```python
from build123d import *

# Parameters (mm, degrees)
F1_DEPTH  = 78.74
F4_W      = 50.8
F4_H      = 25.4
F6_DEPTH  = 11.43
F7_W      = 48.6228571429
F7_H      = 23.7671428571
F10_DEPTH = 3.81
F12_DEPTH = 53.34
F14_DEPTH = 38.1
F16_D     = 6.7564
F16_DEPTH = 7.62
F16_TIP   = 2.0298273432


with BuildPart() as f1:
    # F0 (on Front) → F1 (new body)
    with BuildSketch(Plane.XZ):
        with BuildLine():
            Line((-21.59, 12.7), (-21.59, -12.7))
            ThreePointArc((-21.59, -12.7), (0, -34.29), (21.59, -12.7))
            Line((21.59, -12.7), (21.59, 0))
            Line((21.59, 0), (21.59, 12.7))
            ThreePointArc((21.59, 12.7), (0, 34.29), (-21.59, 12.7))
        make_face()
    extrude(amount=F1_DEPTH)

    # F4 (on Front) → F5 section 0
    with BuildSketch(Plane.XZ):
        with BuildLine():
            Line((-25.4, 12.7), (25.4, 12.7))
            ThreePointArc((25.4, 12.7), (0, 38.1), (-25.4, 12.7))
        make_face()
    # F3 (on offset) → F5 section 1
    with BuildSketch(Plane.XZ.offset(-26.67)):
        with BuildLine():
            Line((-22.86, 8.89), (22.86, 8.89))
            ThreePointArc((22.86, 8.89), (0, 31.75), (-22.86, 8.89))
        make_face()
    loft()

    # F4 (on Front) → F6 (join)
    with BuildSketch(Plane.XZ):
        with BuildLine():
            Line((-25.4, 12.7), (25.4, 12.7))
            ThreePointArc((25.4, 12.7), (0, 38.1), (-25.4, 12.7))
        make_face()
        Rectangle(F4_W, F4_H)
        with BuildLine():
            ThreePointArc((-25.4, -12.7), (0, -38.1), (25.4, -12.7))
            Line((25.4, -12.7), (-25.4, -12.7))
        make_face()
    extrude(amount=-F6_DEPTH)

    # F7 (on face) → F8 section 0
    with BuildSketch(Plane(origin=(0, 11.43, 0), x_dir=(-1, 0, 0), z_dir=(0, 1, 0))):
        with Locations((0, -0.8164285714)):
            Rectangle(F7_W, F7_H)
    # F3 (on offset) → F8 section 1
    with BuildSketch(Plane.XZ.offset(-26.67)):
        with BuildLine():
            ThreePointArc((22.7188888889, 6.3539227823), (22.8246949596, 7.62), (22.86, 8.89))
            Line((22.86, 8.89), (-22.86, 8.89))
            ThreePointArc((-22.86, 8.89), (-22.8245852305, 7.61802946), (-22.7184506514, 6.35))
            Line((-22.7184506514, 6.35), (22.7188888889, 6.3539227823))
        make_face()
    loft()

    # F3 (on offset) → F9 section 0
    with BuildSketch(Plane.XZ.offset(-26.67)):
        with BuildLine():
            ThreePointArc((-22.7184506514, 6.35), (0.0019735927, -13.9699999148), (22.7188888889, 6.3539227823))
            Line((22.7188888889, 6.3539227823), (-22.7184506514, 6.35))
        make_face()
    # F7 (on face) → F9 section 1
    with BuildSketch(Plane(origin=(0, 11.43, 0), x_dir=(-1, 0, 0), z_dir=(0, 1, 0))):
        with BuildLine():
            Line((24.3114285714, -12.7), (-24.3114285714, -12.7))
            ThreePointArc((-24.3114285714, -12.7), (0, -37.0114285714), (24.3114285714, -12.7))
        make_face()
    loft()

    # F3 (on offset) → F10 (join)
    with BuildSketch(Plane.XZ.offset(-26.67)):
        with BuildLine():
            Line((-22.86, 8.89), (22.86, 8.89))
            ThreePointArc((22.86, 8.89), (0, 31.75), (-22.86, 8.89))
        make_face()
        with BuildLine():
            ThreePointArc((22.7188888889, 6.3539227823), (22.8246949596, 7.62), (22.86, 8.89))
            Line((22.86, 8.89), (-22.86, 8.89))
            ThreePointArc((-22.86, 8.89), (-22.8245852305, 7.61802946), (-22.7184506514, 6.35))
            Line((-22.7184506514, 6.35), (22.7188888889, 6.3539227823))
        make_face()
        with BuildLine():
            ThreePointArc((-22.7184506514, 6.35), (0.0019735927, -13.9699999148), (22.7188888889, 6.3539227823))
            Line((22.7188888889, 6.3539227823), (-22.7184506514, 6.35))
        make_face()
    extrude(amount=-F10_DEPTH)

    # F11 (on Front) → F12 (join)
    with BuildSketch(Plane.XZ):
        with BuildLine():
            Line((12.7, 12.7), (12.7, 34.6970452561))
            ThreePointArc((12.7, 34.6970452561), (0, 38.1), (-12.7, 34.6970452561))
            Line((-12.7, 34.6970452561), (-12.7, 12.7))
            Line((-12.7, 12.7), (12.7, 12.7))
        make_face()
    extrude(amount=F12_DEPTH)

    # F13 (on Top) → F14 (join)
    with BuildSketch(Plane.XY):
        Polygon((21.59, -35.56), (21.59, 15.24), (-21.59, 15.24), (-21.59, -35.56), (-8.89, -35.56), (-8.89, -78.74), (8.89, -78.74), (8.89, -35.56), align=None)
    extrude(amount=-F14_DEPTH)

    # F16
    with Locations(Plane(origin=(0, 0, -38.1), x_dir=(1, 0, 0), z_dir=(0, 0, -1))):
        with Locations((0, 55.88)):
            Hole(F16_D / 2, depth=F16_DEPTH)
            with Locations((0, 0, -(F16_DEPTH + F16_TIP / 2))):  # 118° drill point
                Cone(0, F16_D / 2, F16_TIP, mode=Mode.SUBTRACT)


solid = f1.part
```
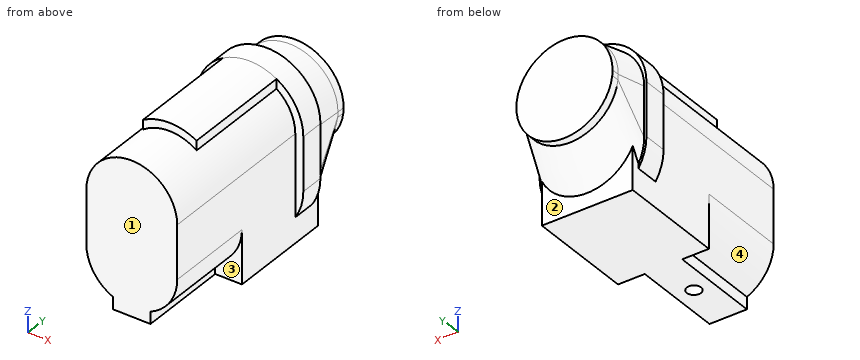
Check sheet for the modelled part. Datum: model origin and axes. Units: mm. Face numbers are marked on the shaded views. A direction names the side the tool comes from. Coordinates: 2 decimals unless noted, no trailing zeros. Write each loop counter-clockwise with the first axis right and the second up, starting at its lowest first coordinate (ties: lowest second). Pieces come first, ordered by that corner, then holes. Notation, with made-up numbers: (42, 1.5) - (59, 1.5) arc R22 ccw to (59, 7.5) - close; hole circle Ø9 at (62.5, 24.5). An arc over 180 degrees is marked (long way). One line per question, with ' | ' between items.
Item 1: Access from +Z, -Z, +X, -X, +Y, -Y to the whole of each face (thin tool, end or side, straight path). Record for the marked faces 1, 2, 3 and 4.
Determined:
face 1: +Z, -Z, +X, -X, -Y | face 2: -Z, +Y | face 3: -Z, +X, -Y | face 4: -Z, -X, -Y
Item 2: Thickness scan on line 1 (X direction, y = -55.88, z = -35.5); line 2 (Y direction, x = 0, z = -32); line 3 (X direction, y = -42, z = 0). Record the ranges inside material, lowest first. Write a range as [from, to].
Determined:
line 1: x = [-8.89, -3.38], [3.38, 8.89] | line 2: y = [-78.74, -59.26], [-52.5, 15.24] | line 3: x = [-21.59, 21.59]
Item 3: Sectioned sample at B-B on y = -26.5. Record the boundary of the cut face in (x, z), plus the area to 3 significant figures.
Determined:
outline: (-21.59, -38.1) - (21.59, -38.1) - (21.59, 12.7) arc R21.59 ccw to (12.7, 30.16) - (12.7, 34.7) arc R25.4 ccw to (-12.7, 34.7) - (-12.7, 30.16) arc R21.59 ccw to (-21.59, 12.7) - close | area: 3,030 mm2
Item 4: Gauge pin test, flat ends, axial feed: P1, Ø8, axis at y = -9.5, z = -16, coming from the +X side; P2, Ø5, axis at y = -31, z = 32.5, coming from the -X side; P3, Ø8, axis at y = 2, z = -17, coming from the +X side. Record the tip position at first contact, or that the pin passes through.
Determined:
P1: stops at x = 21.59 | P2: stops at x = -12.92 | P3: stops at x = 25.4
Item 5: Sectioned sample at A-A on y = -65. Record the boundary of the cut face in (x, z).
Determined:
outline: (-21.59, -12.7) arc R21.59 ccw to (-8.89, -32.37) - (-8.89, -38.1) - (8.89, -38.1) - (8.89, -32.37) arc R21.59 ccw to (21.59, -12.7) - (21.59, 12.7) arc R21.59 ccw to (-21.59, 12.7) - close
